Work out the finished part from the listing and answer in its coordinate system (mm). A direction names the side the tool comes from. Coordinates: 2 decimals unless noted, no trailing zeros. Loops run counter-clockwise (first coordinate to the right, second up) from the corner with the lowest first, then second, coordinate; pieces in that order, holes last. Notation, with made-up numbers: M 24,83 L 31,83 A31 cw 31,114 Z; hole C 68.5,-38 d8. An arc over 180 degrees is marked long. Write each question's results on one line, items separated by ' | '.
```python
from build123d import *

# Parameters (mm, degrees)
BOSS_EXTRUDE1_DEPTH = 200


with BuildPart() as part:
    # Sketch1 → Boss-Extrude1 (new body)
    with BuildSketch(Plane.XY):
        with BuildLine():
            Line((17.715117093, 28.909882907), (12.45, 34.175))
            Line((12.45, 34.175), (12.45, 39))
            Line((12.45, 39), (17.5, 39))
            Line((17.5, 39), (17.5, 43.5))
            Line((17.5, 43.5), (17, 43.5))
            Line((17, 43.5), (17, 45))
            Line((17, 45), (3, 45))
            ThreePointArc((3, 45), (0.878679656, 44.121320344), (0, 42))
            Line((0, 42), (0, 28))
            Line((0, 28), (1.5, 28))
            Line((1.5, 28), (1.5, 27.5))
            Line((1.5, 27.5), (6, 27.5))
            Line((6, 27.5), (6, 32.55))
            Line((6, 32.55), (10.825, 32.55))
            Line((10.825, 32.55), (16.090117093, 27.284882907))
            Line((16.090117093, 27.284882907), (16.090117093, 17.715117093))
            Line((16.090117093, 17.715117093), (10.825, 12.45))
            Line((10.825, 12.45), (6, 12.45))
            Line((6, 12.45), (6, 17.5))
            Line((6, 17.5), (1.5, 17.5))
            Line((1.5, 17.5), (1.5, 17))
            Line((1.5, 17), (0, 17))
            Line((0, 17), (0, 3))
            ThreePointArc((0, 3), (0.878679656, 0.878679656), (3, 0))
            Line((3, 0), (17, 0))
            Line((17, 0), (17, 1.5))
            Line((17, 1.5), (17.5, 1.5))
            Line((17.5, 1.5), (17.5, 6))
            Line((17.5, 6), (12.45, 6))
            Line((12.45, 6), (12.45, 10.825))
            Line((12.45, 10.825), (17.715117093, 16.090117093))
            Line((17.715117093, 16.090117093), (27.284882907, 16.090117093))
            Line((27.284882907, 16.090117093), (32.55, 10.825))
            Line((32.55, 10.825), (32.55, 6))
            Line((32.55, 6), (27.5, 6))
            Line((27.5, 6), (27.5, 1.5))
            Line((27.5, 1.5), (28, 1.5))
            Line((28, 1.5), (28, 0))
            Line((28, 0), (42, 0))
            ThreePointArc((42, 0), (44.121320344, 0.878679656), (45, 3))
            Line((45, 3), (45, 17))
            Line((45, 17), (43.5, 17))
            Line((43.5, 17), (43.5, 17.5))
            Line((43.5, 17.5), (39, 17.5))
            Line((39, 17.5), (39, 12.45))
            Line((39, 12.45), (34.175, 12.45))
            Line((34.175, 12.45), (28.909882907, 17.715117093))
            Line((28.909882907, 17.715117093), (28.909882907, 27.284882907))
            Line((28.909882907, 27.284882907), (34.175, 32.55))
            Line((34.175, 32.55), (39, 32.55))
            Line((39, 32.55), (39, 27.5))
            Line((39, 27.5), (43.5, 27.5))
            Line((43.5, 27.5), (43.5, 28))
            Line((43.5, 28), (45, 28))
            Line((45, 28), (45, 42))
            ThreePointArc((45, 42), (44.121320344, 44.121320344), (42, 45))
            Line((42, 45), (28, 45))
            Line((28, 45), (28, 43.5))
            Line((28, 43.5), (27.5, 43.5))
            Line((27.5, 43.5), (27.5, 39))
            Line((27.5, 39), (32.55, 39))
            Line((32.55, 39), (32.55, 34.175))
            Line((32.55, 34.175), (27.284882907, 28.909882907))
            Line((27.284882907, 28.909882907), (17.715117093, 28.909882907))
        make_face()
    extrude(amount=BOSS_EXTRUDE1_DEPTH)


solid = part.part
```
1) For a pull along X with two mould halves and no side action, classify faces 4 (the face through (23, 28.91, 99)), 5 (the face through (4, 27.5, 99)), 6 (the face through (45, 10, 99)) as released by +X, released by -X, zero draft, split by the parting line, or undercut.
Check result:
face 4: undercut | face 5: zero draft | face 6: released by +X
2) Straight lines are drawn through the part: probe 1 along X at (y, z) = (41.5, 141); probe 2 along Y at (x, z) = (29, 90.5) (3 decimals); probe 3 along X at (y, z) = (7.5, 141). For each, find the intervals that lie inside material, in ascending order. Write a range as [from, to].
Check result:
probe 1: [0, 17.5], [27.5, 45] | probe 2: [0, 6], [14.375, 17.625], [27.375, 30.625], [39, 45] | probe 3: [0, 12.45], [32.55, 45]
3) Find section A-A, the plane x = 22.5. Give the vertices of the cut face in (y, z), and give its area (3 significant figures).
Check result:
outline: M 16.09,0 L 28.91,0 L 28.91,200 L 16.09,200 Z | area: 2,560 mm^2
4) Given pin 1 Ø2 at (x, y) = (33, 17.5) entering from -Z; pin 2 Ø1.6 at (x, z) = (1, 88) entering from +Y; pin 3 Ø0.8 at (y, z) = (44.5, 105) entering from +X, each flat-ended and moving along its own axis, determine where each tip first touches the part or whether it passes through.
Check result:
pin 1: through | pin 2: y = 44.75 | pin 3: x = 44.14
5) Which of the six approach directions +Z, -Z, +X, -X, +Y, -Y give full straight-line access (tool end or side, diameter ignored) to faces 1 (the face through (22, 23, 200)), 2 (the face through (17.5, 4, 99)), 3 (the face through (39, 30, 99))?
Check result:
face 1: +Z, +X, -X, +Y, -Y | face 2: +Z, -Z, -Y | face 3: +Z, -Z
